Could you check a few things on this model? Use its own coordinates, in mm. A direction names the side the tool comes from. Give positions to 0.01 mm unless a question says otherwise; leave off trailing zeros. Loops run counter-clockwise (first coordinate to the right, second up) from the corner with the lowest first, then second, coordinate; pieces in that order, holes last.
1. For faces 4 (the flat face through (-10, -3, 3)), 5 (the cylindrical face through (-5.362, 12.932, -0.007)), which set-ups out of +Z, -Z, +X, -X, +Y, -Y let a thin tool reach every point of the face, with its end or its side?
2. Imagine slicing it at A-A (x = -11.5). List the corners of the cut face in (y, z) for me, plus the area to 3 significant figures.
3. Thinking about a two-plate mould opening in X: for faces 1 (the cylindrical face through (-10, 0, 4)), 2 (the flat face through (-3.3, -3.3, -0.5)), 3 (the cylindrical face through (5.341, -4.656, 2.458)), which applies, +X half, -X half, draft (parallel to the pull), parting line (faces both ways), or undercut?
4. Imagine slicing it at B-B (y = 0). Count the separate pieces of the cut face and the enclosed holes in it, plus the area to 4 significant figures.
5. I need wall thicknesses on line 1 along Z through (x, y) = (-5, 12.5); line 2 along Y through (x, z) = (0, 3.9); line 3 along Y through (x, z) = (5.5, 2.2). Which ranges of each line are inside material? Lowest first, please.
6. Imagine slicing it at C-C (x = 2.75). List the corners of the cut face in (y, z) for me, plus the area to 3 significant figures.
Autodesk Inventor part; units mm, degrees
ref_plane "YZ Plane" through (0, 0, 0) normal (1, 0, 0) x (0, 1, 0)
ref_plane "XZ Plane" through (0, 0, 0) normal (0, 1, 0) x (-1, 0, 0)
ref_plane "XY Plane" through (0, 0, 0) normal (0, 0, 1) x (1, 0, 0)
sketch "Sketch1" plane through (0, 0, 0) normal (1, 0, 0) x (0, 1, 0)
  line L0 (0, 3) -> (14, 3)
  line L1 (14, 3) -> (14, -0.5)
  line L2 (14, -0.5) -> (0, -0.5)
  line L3 (0, -0.5) -> (0, 3)
  line L4 (0, -1.7) -> (0, 6.7)
  line L5 (14, 2) -> (14, 0.5)
  line L6 (14, 0.5) -> (10, 0.5)
  line L7 (10, 0.5) -> (10, 2)
  line L8 (10, 2) -> (14, 2)
  line L9 (10, 3) -> (10, 4.5)
  line L10 (10, 4.5) -> (14, 4.5)
  line L11 (14, 4.5) -> (14, 5.5)
  line L12 (14, 5.5) -> (0, 5.5)
  point P0 (0, 0)
  dimension "d0" = 3.5
  dimension "d1" = 3
  dimension "d2" = 14
  dimension "d4" = 1
  dimension "d5" = 1
  dimension "d19" = 4
  dimension "d26" = 1.5
  dimension "d27" = 1
revolve "Revolution1" add sketch "Sketch1" angle 360 about axis through (0, 0, -10) along (0, 0, 1) contours L4 L12 L11 L10 L9 L0 | L0 L1 L8 L7 L6 L2 L3
sketch "Sketch2" plane through (0, 0, -0.5) normal (0, 0, -1) x (-1, 0, 0)
  circle A0 centre (0, 8) radius 1.05
  circle A1 centre (0, 0) radius 4.5
  dimension "d7" = 2.1
  dimension "d8" = 8
  dimension "d9" = 9
extrude "Extrusion1" cut sketch "Sketch2" against normal blind 100
pattern_circular "Circular Pattern1" count 8 over 360 about axis through (0, 0, -10) along (0, 0, 1) of "Extrusion1"
sketch "Sketch3" plane through (0, 0, -0.5) normal (0, 0, -1) x (-1, 0, 0)
  circle A0 centre (-10, 0) radius 1.25
  circle A1 centre (-8, 0) radius 1.05
  point P0 (0, 0)
  point P1 (-8.885, -0.565)
  point P2 (-8.885, 0.565)
  dimension "d15" = 2.5
  dimension "d16" = 10
extrude "Extrusion2" add sketch "Sketch3" against normal blind 6
extrude "Extrusion5" cut sketch "Sketch3" against normal blind 100 contours A0 A1 | A1 A0 picked at (-8.9455, 0) picked at (-10.5022, 0.1399)
properties part number "Motor_pulley"
Derived:
1. face 4: none
1. face 5: +Z, -Z
2. outline: (-7.98, -0.5) - (7.98, -0.5) - (7.98, 0.5) - (-7.98, 0.5) - close; (-7.98, 2) - (7.98, 2) - (7.98, 3) - (-7.98, 3) - close; (-7.98, 4.5) - (7.98, 4.5) - (7.98, 5.5) - (-7.98, 5.5) - close
2. area: 47.9 mm2
3. face 1: parting line
3. face 2: draft
3. face 3: undercut
4. separate pieces: 6
4. enclosed holes: 0
4. area: 66.15 mm2
5. line 1: z = -0.5 to 0.5, 2 to 3, 4.5 to 5.5
5. line 2: y = -10 to -9.05, -6.95 to -4.5, 4.5 to 6.95, 9.05 to 10
5. line 3: y = -12.87 to -6.7, -4.62 to 4.62, 6.7 to 12.87
6. outline: (-13.73, -0.5) - (-3.56, -0.5) - (-3.56, 5.5) - (-13.73, 5.5) - (-13.73, 4.5) - (-9.61, 4.5) - (-9.61, 3) - (-13.73, 3) - (-13.73, 2) - (-9.61, 2) - (-9.61, 0.5) - (-13.73, 0.5) - close; (3.56, -0.5) - (13.73, -0.5) - (13.73, 0.5) - (9.61, 0.5) - (9.61, 2) - (13.73, 2) - (13.73, 3) - (9.61, 3) - (9.61, 4.5) - (13.73, 4.5) - (13.73, 5.5) - (3.56, 5.5) - close
6. area: 97.3 mm2
